Verification items for the finished model (mm, model axes). A direction names the side the tool comes from. Round coordinates to 2 decimals unless told otherwise and drop trailing zeros. Loops run counter-clockwise (first coordinate to the right, second up) from the corner with the lowest first, then second, coordinate; pieces in that order, holes last. Notation, with made-up numbers: (56.25, 1.5) -> (86.25, 1.5) arc R14 ccw to (86.25, 28.5) -> close; hole circle Ø2 at (13.5, 59.5). An arc over 180 degrees is marked (long way). Write item = value, one per line.
Solid Edge part; units mm, degrees
sketch "Sketch1" plane through (0, 0, 0) normal (0, -1, 0) x (1, 0, 0)
  line L0 (-5.3694, 18.9) -> (-19.0694, -4.8291)
  arc A0 (-13.7, -14.1291) -> (-19.0694, -4.8291) centre (-13.7, -7.9291) cw
  line L1 (-13.7, -14.1291) -> (13.7, -14.1291)
  arc A1 (19.0694, -4.8291) -> (13.7, -14.1291) centre (13.7, -7.9291) cw
  line L2 (5.3694, 18.9) -> (19.0694, -4.8291)
  arc A2 (-5.3694, 18.9) -> (5.3694, 18.9) centre (0, 15.8) cw
  dimension "D1" = 5.3694
extrude "Protrusion1" add sketch "Sketch1" against normal blind 16
sketch "Sketch2" plane through (0, 0, 0) normal (0, -1, 0) x (1, 0, 0)
  circle A0 centre (-13.7, -7.9291) radius 2.2
  circle A1 centre (13.7, -7.9291) radius 2.2
  circle A2 centre (0, 15.8) radius 2.2
extrude "Cutout1" cut sketch "Sketch2" against normal blind 457.8755
sketch "Sketch3" plane through (0, 0, 0) normal (0, -1, 0) x (1, 0, 0)
  circle A0 centre (0, 0) radius 8.2
extrude "Cutout2" cut sketch "Sketch3" against normal blind 434.4917
sketch "Sketch4" plane through (0, 0, 3.9355) normal (0, -1, 0) x (-0.5, 0, 0.866)
  line L0 (-23.325, -5.9323) -> (-23.325, -18.9323)
  line L1 (-23.325, -18.9323) -> (16.475, -18.9323)
  line L2 (16.475, -18.9323) -> (16.475, -5.9323)
  line L3 (12.7755, -8.7037) -> (16.475, -5.9323)
  line L4 (-20.9306, -8.7037) -> (12.7755, -8.7037)
  line L5 (-20.9306, -5.9323) -> (-20.9306, -8.7037)
  line L6 (-23.325, -5.9323) -> (-20.9306, -5.9323)
  dimension "D1" = 23.325
extrude "Protrusion2" add sketch "Sketch4" against normal up to vertex (16 mm away)
sketch "Sketch5" plane through (3.1086, 0, 6.2098) normal (0, -1, 0) x (-0.5, 0, 0.866)
  line L0 (-10.3403, 2.4623) -> (-10.3403, -10.1029)
  line L1 (-10.3403, -10.1029) -> (2.6597, -10.1029)
  line L2 (2.6597, -10.1029) -> (2.6597, 2.4623)
  line L3 (2.6597, 2.4623) -> (-10.3403, 2.4623)
extrude "ExtrudedCutout_18" cut sketch "Sketch5" against normal blind 196.9446
sketch "Sketch6" plane through (13.7782, 8, 7.9355) normal (-0.866, 0, -0.5) x (0, -1, 0)
  line L0 (-2, 3.4641) -> (2, 3.4641)
  line L1 (-4, 0) -> (-2, 3.4641)
  line L2 (-2, -3.4641) -> (-4, 0)
  line L3 (2, -3.4641) -> (-2, -3.4641)
  line L4 (5.4641, 0) -> (2, -3.4641)
  line L5 (2, 3.4641) -> (5.4641, 0)
extrude "ExtrudedCutout_19" cut sketch "Sketch6" against normal blind 4
sketch "Sketch7" plane through (18.1083, 8, 10.4355) normal (0.866, 0, 0.5) x (-0.5, 0, 0.866)
  line L0 (-19.9, 8) -> (19.9, 8)
  line L1 (19.9, -8) -> (19.9, 8)
  line L2 (-19.9, -8) -> (19.9, -8)
  line L3 (-19.9, -8) -> (-19.9, 8)
extrude "ExtrudedProtrusion_14" add sketch "Sketch7" along normal blind 4
sketch "Sketch8" plane through (21.5724, 8, 12.4355) normal (0.866, 0, 0.5) x (-0.5, 0, 0.866)
  line L0 (-1.5556, 1.5556) -> (0, 3.1113)
  line L1 (0, 3.1113) -> (1.5556, 1.5556)
  arc A0 (1.5556, 1.5556) -> (-1.5556, 1.5556) centre (0, 0) cw
extrude "ExtrudedCutout_20" cut sketch "Sketch8" against normal blind 25.1595
(1) Sectioned sample at B-B, the plane y = 11. Count the separate pieces of the cut face and the enclosed holes in it, and give its area (3 significant figures).
Filled sheet:
separate_pieces = 1
enclosed_holes = 4
area = 1,020 mm2
(2) Go/stop test with flat-tipped pins: pin 1 Ø1.5 at (y, z) = (11, 2.5) entering from -X; pin 2 Ø3 at (y, z) = (9.5, 4.5) entering from -X; pin 3 Ø6 at (x, y) = (17, 8.5) entering from -Z. Record where each tip stops, or that it passes through.
Filled sheet:
pin_1 = -15.27
pin_2 = -14.55
pin_3 = -14.12
(3) Draft check along Z on faces 4 (the face through (-19.114, 7.888, -10.95)), 5 (the face through (9.866, 8.112, 28.655)), 6 (the face through (14.61, 4.29, 10.44)). Enter one of: released by +Z, released by -Z, zero draft, split by the parting line, or undercut.
Filled sheet:
face_4 = split by the parting line
face_5 = released by +Z
face_6 = undercut
(4) Sectioned sample at A-A, the plane z = -0.5. Record the cut outline in (x, y).
Filled sheet:
outline = (-16.57, 0) -> (-8.18, 0) -> (-8.18, 16) -> (-16.57, 16) -> close; (12.17, 0) -> (29.04, 0) -> (29.04, 16) -> (12.17, 16) -> close
(5) Material ranges on probe 1 along Z at (x, y) = (0, 4.25); probe 2 along Z at (x, y) = (-0.5, 2); probe 3 along Z at (x, y) = (10.5, 14.25), recorded low to high. Write a range as from..to.
Filled sheet:
probe_1 = -14.13..-8.2, 8.2..13.6, 18..22.96
probe_2 = -14.13..-8.18, 8.18..13.66, 17.94..22.67
probe_3 = -14.13..-1.46, 13.55..29.02
(6) Set-up check for faces 1 (the face through (12.232, 7.888, -0.463)), 2 (the face through (-12.123, 7.888, 7.202)), 3 (the face through (14.632, 11.014, 10.4)): record each of +Z, -Z, +X, -X, +Y, -Y from which the full face is reachable in a straight line by a thin tool's end or side.
Filled sheet:
face_1 = +Y, -Y
face_2 = +Z, -X, +Y, -Y
face_3 = none
(7) Sectioned sample at C-C, the plane z = 15.8. Record the cut outline in (x, y), and give its area (3 significant figures).
Filled sheet:
outline = (-7.16, 0) -> (-2.2, 0) -> (-2.2, 16) -> (-7.16, 16) -> close; (2.2, 0) -> (19.63, 0) -> (19.63, 16) -> (2.2, 16) -> close
area = 358 mm2
(8) Sectioned sample at D-D, the plane x = -10. Record the cut outline in (y, z), and give its area (3 significant figures).
Filled sheet:
outline = (0, -14.13) -> (16, -14.13) -> (16, 10.88) -> (0, 10.88) -> close
area = 400 mm2
